The listing builds one solid part. Answer for the finished solid, in the listing's coordinates (mm). A direction names the side the tool comes from. Give positions to 0.01 mm unless a question says otherwise; leave off trailing zeros. Order: outer loops, then holes, each group sorted by start corner. A loop starts at its lowest first (then second) coordinate and runs counter-clockwise, first axis right, second up. Notation, with made-up numbers: (-1, 41) - (40, 41) arc R26 ccw to (40, 74) - close; hole circle Ø10 at (53, -38.5). An arc over 180 degrees is marked (long way). Use a Markdown table: item, result. Add a question column.
1) Find section A-A, the plane x = 0. Determine the outline of the cut face in (y, z).
2) Straight lines are drawn through the part: line 1 (Y direction, x = 0, z = 4); line 2 (Z direction, x = -2.5, y = -2.5); line 3 (X direction, y = 2.5, z = 5.25). For each, find the intervals that lie inside material, in ascending order.
3) The mould has two halves that part along Y. Classify faces 1 (the face through (0, 0, 0)), 2 (the face through (-1, 38.1, 0)), 3 (the face through (8, 1, 6.35)): released by +Y, released by -Y, zero draft, split by the parting line, or undercut.
4) Find section B-B, the plane z = 4.25. Determine the outline of the cut face in (x, y), plus the area to 3 significant figures.
5) For faces 4 (the face through (-1.38, -6.2, 3.22)), 5 (the face through (-38.1, -1, 0)), determine the directions among +Z, -Z, +X, -X, +Y, -Y from which every point of the face is accessible in a straight line to the end or side of a thin tool.
from build123d import *

# Parameters (mm, degrees)
F0_W     = 76.2
F0_H     = 76.2
F1_DEPTH = 6.35
F2_R     = 6.35
F3_DEPTH = 6.35


with BuildPart() as f1:
    # F0 (on Top) → F1 (new body, symmetric)
    with BuildSketch(Plane.XY):
        Rectangle(F0_W, F0_H)
    extrude(amount=F1_DEPTH, both=True)

    # F2 (on face) → F3 (cut)
    with BuildSketch(Plane.XY.offset(6.35)):
        Circle(F2_R)
    extrude(amount=-F3_DEPTH, mode=Mode.SUBTRACT)


solid = f1.part
The answers:
| question | item | result |
|---|---|---|
| 1 | outline | (-38.1, -6.35) - (38.1, -6.35) - (38.1, 6.35) - (6.35, 6.35) - (6.35, 0) - (-6.35, 0) - (-6.35, 6.35) - (-38.1, 6.35) - close |
| 2 | line 1 | -38.1 to -6.35, 6.35 to 38.1 |
| 2 | line 2 | -6.35 to 0 |
| 2 | line 3 | -38.1 to -5.84, 5.84 to 38.1 |
| 3 | face 1 | undercut |
| 3 | face 2 | released by +Y |
| 3 | face 3 | zero draft |
| 4 | outline | (-38.1, -38.1) - (38.1, -38.1) - (38.1, 38.1) - (-38.1, 38.1) - close; hole circle Ø12.7 at (0, 0) |
| 4 | area | 5,680 mm2 |
| 5 | face 4 | +Z |
| 5 | face 5 | +Z, -Z, -X, +Y, -Y |
